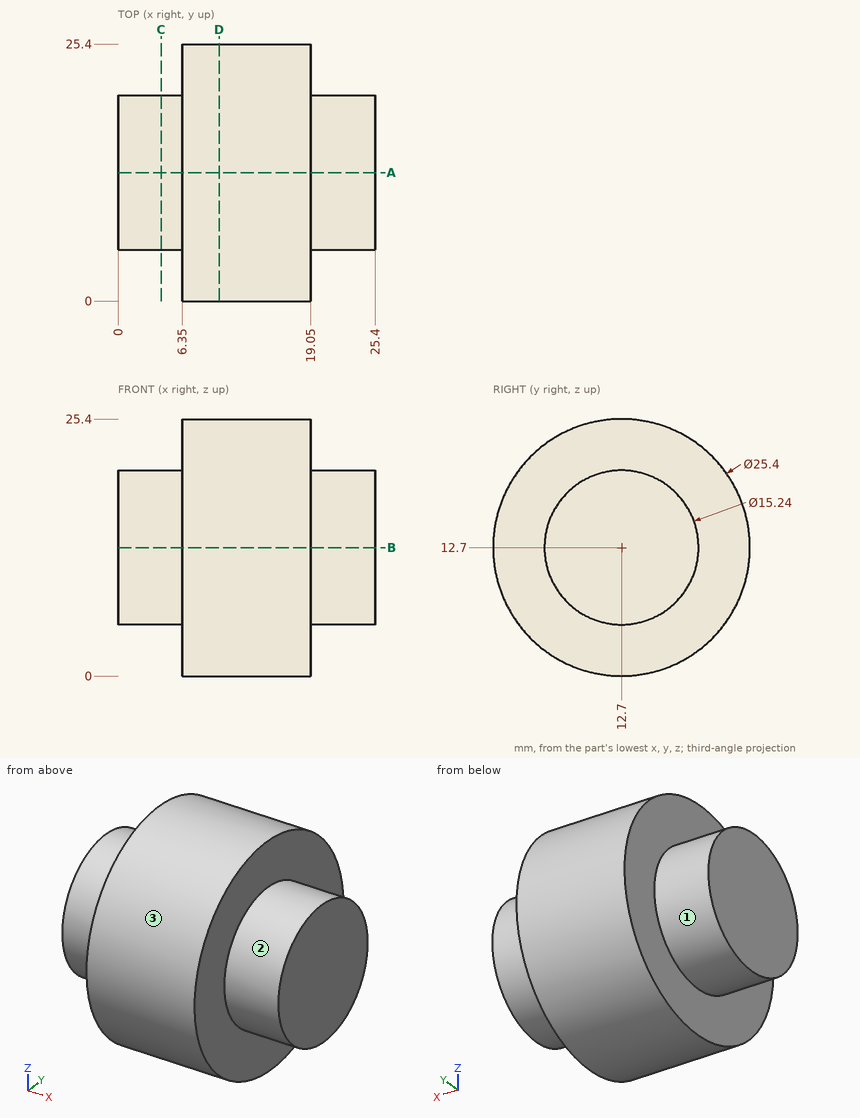
Geometry: see drawing. Coordinates: mm, zero at the bounding-box minimum. A direction names the side the tool comes from. Give positions to 0.01 mm unless a question says otherwise; leave off trailing zeros. Loops run counter-clockwise (first coordinate to the right, second up) from the corner with the lowest first, then second, coordinate; pieces in that order, holes last. Notation, with made-up numbers: (56, 78) -> (108, 78) arc R16 cw to (108, 91) -> close; hole circle Ø5 at (42.25, -29). An arc over 180 degrees is marked (long way). Answer as a JSON object with one key per item and string values. Group by question number.
Item 1: Cut plane C-C, the plane x = 4.25. Return the cut outline in (y, z), and give its area (3 significant figures).
Item 2: Line query: probe 1 along X at (y, z) = (13.5, 4.75); probe 2 along Z at (x, y) = (21, 12.5); probe 3 along Y at (x, z) = (10.75, 12.5). Output: solid intervals per line, ascending.
Item 3: Cut plane D-D, the plane x = 10. Return the cut outline in (y, z), and give its area (3 significant figures).
Item 4: Reachability of the marked faces 1, 2 and 3 from +Z, -Z, +X, -X, +Y, -Y: full face, straight path, thin tool, end or side. Return the list, or none.
Item 5: Cut plane A-A, the plane y = 12.7. Return the cut outline in (x, z), and give its area (3 significant figures).
Item 6: Pin query (flat end, axial travel): P1, Ø1.5, axis at x = 8.5, y = 5, coming from the +Z side; P2, Ø3, axis at x = 21, y = 20, coming from the +Z side; P3, Ø12, axis at x = 10, y = 22, coming from the +Z side. Return the tip coordinate at first contact, or that it passes through.
Checks:
{
 "1": {"outline": "circle Ø15.24 at (12.7, 12.7)", "area": "182 mm²"},
 "2": {"probe 1": "x = 6.35 to 19.05", "probe 2": "z = 5.08 to 20.32", "probe 3": "y = 0 to 25.4"},
 "3": {"outline": "circle Ø25.4 at (12.7, 12.7)", "area": "507 mm²"},
 "4": {"face 1": "-X", "face 2": "+X", "face 3": "+X, -X"},
 "5": {"outline": "(0, 5.08) -> (6.35, 5.08) -> (6.35, 0) -> (19.05, 0) -> (19.05, 5.08) -> (25.4, 5.08) -> (25.4, 20.32) -> (19.05, 20.32) -> (19.05, 25.4) -> (6.35, 25.4) -> (6.35, 20.32) -> (0, 20.32) -> close", "area": "516 mm²"},
 "6": {"P1": "stops at z = 23.33", "P2": "stops at z = 17.64", "P3": "stops at z = 24.96"}
}
